Source: CAD feature listing. Evaluate the final solid. Frame: model axes, mm. Face numbers are marked on the shaded views. A direction names the side the tool comes from. Coordinates: 2 decimals unless noted, no trailing zeros. Order: outer loops, then holes, each group sorted by start corner. A loop starts at its lowest first (then second) coordinate and runs counter-clockwise, first axis right, second up. Notation, with made-up numbers: (65, 68) - (102, 68) arc R27 cw to (102, 107) - close; hole circle Ø1 at (48.25, 6). An arc over 180 degrees is marked (long way). One line per question, with ' | ' between items.
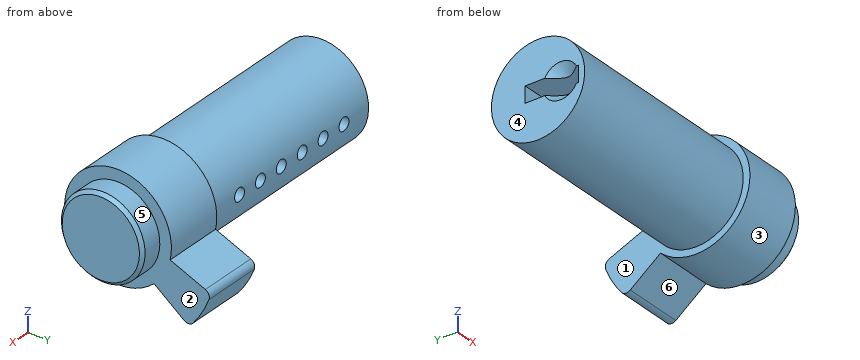
from build123d import *

# Parameters (mm, degrees)
SKETCH1_R           = 7.25
OUTSIDE_DIA_DEPTH   = 32.25
SKETCH2_W           = 2.5
SKETCH2_H           = 8.25
KEYHOLE_DEPTH       = 33.25
SKETCH3_R           = 1
PIN_1_DEPTH         = 35
LPATTERN1_COUNT     = 6
LPATTERN1_PITCH     = 4.25
CAM_DEPTH           = 9.25
FILLET_R1_R         = 1
SKETCH6_R           = 6.5
END_BIT_DEPTH       = 3.5
F_0_5_X_45_DEG_SIZE = 0.5


with BuildPart() as part:
    # Sketch1 → outside dia (new body)
    with BuildSketch(Plane(origin=(0, 0, 0), x_dir=(0, 0, -1), z_dir=(1, 0, 0))):
        Circle(SKETCH1_R)
    extrude(amount=OUTSIDE_DIA_DEPTH)

    # Sketch2 → keyhole (cut, through all)
    with BuildSketch(Plane.ZY):
        with Locations((0, -2.125)):
            Rectangle(SKETCH2_W, SKETCH2_H)
    extrude(amount=-KEYHOLE_DEPTH, mode=Mode.SUBTRACT)

    # Sketch3 → pin 1 (cut)
    with BuildSketch(Plane(origin=(0, 0, 0), x_dir=(1, 0, 0), z_dir=(0, 1, 0))):
        with Locations((5, 0)):
            Circle(SKETCH3_R)
    pin_1 = extrude(amount=PIN_1_DEPTH, mode=Mode.SUBTRACT)

    # LPattern1: pin 1 ×6
    with Locations(*[(i * LPATTERN1_PITCH, 0, 0) for i in range(1, LPATTERN1_COUNT)]):
        add(pin_1, mode=Mode.SUBTRACT)

    # Sketch4 → front cone 5.5 x 90 deg (revolve, cut)
    with BuildSketch(Plane.XY):
        Polygon((0, -3.5), (0, -6.25), (2.75, -3.5), align=None)
    revolve(axis=Axis((2.75, -3.5, 0), (-1, 0, 0)), mode=Mode.SUBTRACT)

    # Sketch5 → cam (add)
    with BuildSketch(Plane(origin=(32.25, 0, 0), x_dir=(0, 0, -1), z_dir=(1, 0, 0))):
        with BuildLine():
            Line((4.411633528, 14.441173415), (1.787227075, 8.105295762))
            ThreePointArc((1.787227075, 8.105295762), (-4.15, -7.188010851), (6.125778497, 5.60043193))
            Line((6.125778497, 5.60043193), (10.300606274, 11.041173415))
            ThreePointArc((10.300606274, 11.041173415), (7.55, 13.076983597), (4.411633528, 14.441173415))
        make_face()
    extrude(amount=CAM_DEPTH)

    # Fillet R1
    fillet_r1_edges = [part.edges().sort_by_distance(p)[0] for p in [
        (36.875, 11.041173415, -10.300606274),
        (36.875, 14.441173415, -4.411633528),
    ]]
    fillet(fillet_r1_edges, radius=FILLET_R1_R)

    # Sketch6 → end bit (add)
    with BuildSketch(Plane(origin=(41.5, 0, 0), x_dir=(0, 0, -1), z_dir=(1, 0, 0))):
        Circle(SKETCH6_R)
    extrude(amount=END_BIT_DEPTH)

    # 0.5 x 45 deg
    f_0_5_x_45_deg_edges = [part.edges().sort_by_distance(p)[0] for p in [
        (45, 0, 6.5),
    ]]
    chamfer(f_0_5_x_45_deg_edges, length=F_0_5_X_45_DEG_SIZE)


solid = part.part
(1) Cut plane B-B (x = 39.5). Return the cut outline in (y, z), and give its area (3 significant figures).
Taken from the geometry:
outline: (5.6, -6.13) - (10.3, -9.73) arc R1 ccw to (11.68, -9.57) arc R15.1 ccw to (14.13, -5.33) arc R1 ccw to (13.58, -4.05) - (8.11, -1.79) arc R8.3 ccw (long way) to start | area: 257 mm²
(2) Cut plane C-C (z = 0). State how many separate pieces and enclosed holes the cut face has, and give its area (3 significant figures).
Taken from the geometry:
separate pieces: 7 | enclosed holes: 0 | area: 337 mm²
(3) Material intervals for L1, parallel to Y at x = 39, z = -6.5; L2, parallel to X at y = 9.5, z = -7.5; L3, parallel to Z at x = 17.5, y = -4, sorted ascending. Write a range as from..to.
Taken from the geometry:
L1: y = -5.16..5.16, 6.09..13.63 | L2: x = 32.25..41.5 | L3: z = -6.05..-1.25, 1.25..6.05
(4) Set-up query: the marked faces 1, 2 and 3. Return all of +Z, -Z, +X, -X, +Y, -Y with unobstructed straight access to the full face (end or side cutting, diameter ignored); none if empty.
Taken from the geometry:
face 1: -X | face 2: +X | face 3: +X, -X
(5) Pin query (flat end, axial travel): P1, Ø4, axis at x = 11.5, y = -1, coming from the -Z side; P2, Ø1, axis at x = 25.5, y = 2, coming from the +Z side; P3, Ø1.2, axis at x = 21.5, z = 0.5, coming from the +Y side. Return the tip coordinate at first contact, or that it passes through.
Taken from the geometry:
P1: stops at z = -7.25 | P2: stops at z = 7.09 | P3: stops at y = 7.25
(6) Cut plane A-A (y = 0). Return the cut outline in (x, z).
Taken from the geometry:
outline: (0, -7.25) - (32.25, -7.25) - (32.25, -8.3) - (41.5, -8.3) - (41.5, -6.5) - (44.5, -6.5) - (45, -6) - (45, 6) - (44.5, 6.5) - (41.5, 6.5) - (41.5, 8.3) - (32.25, 8.3) - (32.25, 7.25) - (0, 7.25) - (0, 1.25) - (32.25, 1.25) - (32.25, -1.25) - (0, -1.25) - close
(7) Pull-direction query (Y, two-part tool) for the marked faces 4, 5 and 6; classes: pulls with the +Y half, pulls with the -Y half, needs draft (parallel to the pull), parting line crosses it, or undercut.
Taken from the geometry:
face 4: needs draft | face 5: parting line crosses it | face 6: undercut
